from build123d import *

# Parameters (mm, degrees)
F0_R     = 32.5
F1_DEPTH = 26
F3_DEPTH = 14.7
F4_R     = 26.5
F5_DEPTH = 9
F7_DEPTH = 25


with BuildPart() as f1:
    # F0 (on Top) → F1 (new body)
    with BuildSketch(Plane.XY):
        Circle(F0_R)
    extrude(amount=F1_DEPTH)

    # F2 (on face) → F3 (cut)
    with BuildSketch(Plane.XY.offset(26)):
        Polygon((-6.544173, 2.2746), (-5.241948, -4.53012), (1.302225, -6.80472), (6.544173, -2.2746), (5.241948, 4.53012), (-1.302225, 6.80472), align=None)
    extrude(amount=-F3_DEPTH, mode=Mode.SUBTRACT)

    # F4 (on face) → F5 (cut)
    with BuildSketch(Plane.XY.offset(26)):
        Circle(F4_R)
    extrude(amount=-F5_DEPTH, mode=Mode.SUBTRACT)

    # F6 (on face) → F7 (cut)
    with BuildSketch(Plane.XY.offset(17)):
        with BuildLine():
            Line((-22.338205, 10.185808), (-8.534389, 3.891523))
            ThreePointArc((-8.534389, 3.891523), (-7.728976, 5.314383), (-6.688723, 6.575768))
            Line((-6.688723, 6.575768), (-17.507295, 17.211645))
            ThreePointArc((-17.507295, 17.211645), (-20.230091, 13.910051), (-22.338205, 10.185808))
        make_face()
        with BuildLine():
            Line((-23.659369, -6.55594), (-9.039144, -2.50472))
            ThreePointArc((-9.039144, -2.50472), (-9.336759, -0.897036), (-9.350681, 0.737903))
            Line((-9.350681, 0.737903), (-24.474798, 1.931412))
            ThreePointArc((-24.474798, 1.931412), (-24.438357, -2.347934), (-23.659369, -6.55594))
        make_face()
        with BuildLine():
            Line((-13.910051, -20.230091), (-5.314383, -7.728976))
            ThreePointArc((-5.314383, -7.728976), (-6.575768, -6.688723), (-7.637352, -5.445236))
            Line((-7.637352, -5.445236), (-19.990271, -14.252549))
            ThreePointArc((-19.990271, -14.252549), (-17.211645, -17.507295), (-13.910051, -20.230091))
        make_face()
        with BuildLine():
            Line((2.347934, -24.438357), (0.897036, -9.336759))
            ThreePointArc((0.897036, -9.336759), (-0.737903, -9.350681), (-2.350421, -9.080488))
            Line((-2.350421, -9.080488), (-6.152074, -23.767585))
            ThreePointArc((-6.152074, -23.767585), (-1.931412, -24.474798), (2.347934, -24.438357))
        make_face()
        with BuildLine():
            Line((17.507295, -17.211645), (6.688723, -6.575768))
            ThreePointArc((6.688723, -6.575768), (5.445236, -7.637352), (4.036298, -8.466879))
            Line((4.036298, -8.466879), (10.564747, -22.161503))
            ThreePointArc((10.564747, -22.161503), (14.252549, -19.990271), (17.507295, -17.211645))
        make_face()
        with BuildLine():
            Line((24.474798, -1.931412), (9.350681, -0.737903))
            ThreePointArc((9.350681, -0.737903), (9.080488, -2.350421), (8.534389, -3.891523))
            Line((8.534389, -3.891523), (22.338205, -10.185808))
            ThreePointArc((22.338205, -10.185808), (23.767585, -6.152074), (24.474798, -1.931412))
        make_face()
        with BuildLine():
            Line((19.990271, 14.252549), (7.637352, 5.445236))
            ThreePointArc((7.637352, 5.445236), (8.466879, 4.036298), (9.039144, 2.50472))
            Line((9.039144, 2.50472), (23.659369, 6.55594))
            ThreePointArc((23.659369, 6.55594), (22.161503, 10.564747), (19.990271, 14.252549))
        make_face()
        with BuildLine():
            Line((6.152074, 23.767585), (2.350421, 9.080488))
            ThreePointArc((2.350421, 9.080488), (3.891523, 8.534389), (5.314383, 7.728976))
            Line((5.314383, 7.728976), (13.910051, 20.230091))
            ThreePointArc((13.910051, 20.230091), (10.185808, 22.338205), (6.152074, 23.767585))
        make_face()
        with BuildLine():
            Line((-0.897036, 9.336759), (-2.347934, 24.438357))
            ThreePointArc((-2.347934, 24.438357), (-6.55594, 23.659369), (-10.564747, 22.161503))
            Line((-10.564747, 22.161503), (-4.036298, 8.466879))
            ThreePointArc((-4.036298, 8.466879), (-2.50472, 9.039144), (-0.897036, 9.336759))
        make_face()
    extrude(amount=-F7_DEPTH, mode=Mode.SUBTRACT)


solid = f1.part
The listing builds one solid part. Answer for the finished solid, in the listing's coordinates (mm). A direction names the side the tool comes from. Coordinates: 2 decimals unless noted, no trailing zeros. Loops run counter-clockwise (first coordinate to the right, second up) from the corner with the lowest first, then second, coordinate; pieces in that order, holes last.
1) Flat-ended cylindrical pins translate along their axes: pin 1 Ø8 at (y, z) = (8, 12) entering from +X; pin 2 Ø8 at (x, y) = (-10.5, 0) entering from +Z; pin 3 Ø6 at (y, z) = (-4, 6) entering from -X. Find the tip coordinate at first contact, or state that the pin passes through.
2) Find section B-B on x = 21. Write down the section's boundary in (y, z).
3) Find section D-D on y = -18.5. Write down the section's boundary in (x, z), then the cut area to 3 significant figures.
4) Find section A-A on y = 13. Write down the section's boundary in (x, z).
5) A tool of negligible diameter and unlimited length cuts with its end or side. For faces 1 (the face through (0, 0, 11.3)), 2 (the face through (-20.196, 13.959, 8.619)), from which of +Z, -Z, +X, -X, +Y, -Y can it reach the whole face along a straight path? Write none if from no direction.
6) Find the intervals of material crossed by L1, parallel to Y at x = 0, z = 21.5; L2, parallel to Y at x = 9.5, z = 13.75; L3, parallel to X at y = -10.5, z = 10.5, in increasing order.
7) Find section C-C on x = 0. Write down the section's boundary in (y, z), then the cut area to 3 significant figures.
Values:
1. pin 1: stops at x = 32.25
1. pin 2: stops at z = 17
1. pin 3: stops at x = -32.48
2. outline: (-24.8, 0) - (-9.58, 0) - (-9.58, 17) - (-16.16, 17) - (-16.16, 26) - (-24.8, 26) - close; (-1.66, 0) - (5.82, 0) - (5.82, 17) - (-1.66, 17) - close; (12.72, 0) - (24.8, 0) - (24.8, 26) - (16.16, 26) - (16.16, 17) - (12.72, 17) - close
3. outline: (-26.72, 0) - (-16.14, 0) - (-16.14, 17) - (-18.97, 17) - (-18.97, 26) - (-26.72, 26) - close; (-12.72, 0) - (-4.79, 0) - (-4.79, 17) - (-12.72, 17) - close; (1.78, 0) - (8.82, 0) - (8.82, 17) - (1.78, 17) - close; (16.14, 0) - (26.72, 0) - (26.72, 26) - (18.97, 26) - (18.97, 17) - (16.14, 17) - close
3. area: 754 mm2
4. outline: (-29.79, 0) - (-20.83, 0) - (-20.83, 17) - (-23.09, 17) - (-23.09, 26) - (-29.79, 26) - close; (-13.22, 0) - (-6.2, 0) - (-6.2, 17) - (-13.22, 17) - close; (-1.25, 0) - (3.36, 0) - (3.36, 17) - (-1.25, 17) - close; (8.94, 0) - (18.23, 0) - (18.23, 17) - (8.94, 17) - close; (20.83, 0) - (29.79, 0) - (29.79, 26) - (23.09, 26) - (23.09, 17) - (20.83, 17) - close
5. face 1: +Z
5. face 2: +Z, -Z
6. L1: y = -32.5 to -26.5, 26.5 to 32.5
6. L2: y = -31.08 to -19.93, -9.34 to -4.33, -0.75 to 2.63, 6.77 to 13.82, 22.64 to 31.08
6. L3: x = -30.76 to -14.73, -7.22 to -2.72, 1.01 to 5.01, 10.68 to 30.76
7. outline: (-32.5, 0) - (-24.55, 0) - (-24.55, 17) - (-26.5, 17) - (-26.5, 26) - (-32.5, 26) - close; (-9.38, 0) - (32.5, 0) - (32.5, 26) - (26.5, 26) - (26.5, 17) - (6.35, 17) - (6.35, 11.3) - (-6.35, 11.3) - (-6.35, 17) - (-9.38, 17) - close
7. area: 883 mm2
